The listing builds one solid part. Answer for the finished solid, in the listing's coordinates (mm). Face numbers are marked on the shaded views. A direction names the side the tool comes from. Coordinates: 2 decimals unless noted, no trailing zeros. Order: outer loops, then holes, each group sorted by start corner. A loop starts at its lowest first (then second) coordinate and runs counter-clockwise, first axis right, second up. Notation, with made-up numbers: M -16.75,-28 L 33.25,-28 A16 ccw 33.25,-9 Z; hole C -1,-16 d6. An arc over 180 degrees is marked long. One line per item, written item: value. Start each with the question number.
Q1. Each of these flat-tipped pins is pushed along its axis until it touches: pin 1 Ø11.5 at (x, z) = (-63.5, 63.5) entering from -Y (3 decimals); pin 2 Ø4 at (x, y) = (-75.5, -5.5) entering from +Z (3 decimals); pin 3 Ø15 at (y, z) = (63.5, 25.4) entering from +X (3 decimals). Where does it stop, or does it pass through?
Q2. The part is cut by section C-C on x = -63.5. Give the vertices of the cut face in (y, z) (3 decimals), then the cut area to 3 significant figures.
Q3. Straight lines are drawn through the part: line 1 along X through (y, z) = (-120, 63); line 2 along Y through (x, z) = (-113, 47) (3 decimals); line 3 along X through (y, z) = (-81, 81) (3 decimals). For each, find the intervals that lie inside material, in ascending order. Write a range as [from, to].
Q4. The part is cut by section B-B on z = 25.4. Give the vertices of the cut face in (x, y) (3 decimals), then the cut area to 3 significant figures.
Q5. Determine the mould class of the marked faces 4, 5, 6 and 7 for opening direction X: pulls with the +X half, pulls with the -X half, needs draft (parallel to the pull), parting line crosses it, or undercut.
Q6. The part is cut by section D-D on z = 127.5. Give the vertices of the cut face in (x, y) (3 decimals).
Q7. The part is cut by section A-A on y = 63.5. Give the vertices of the cut face in (x, z) (3 decimals), then the cut area to 3 significant figures.
Q8. For the marked faces 1, 2 and 3, determine the directions among +Z, -Z, +X, -X, +Y, -Y from which every point of the face is accessible in a straight line to the end or side of a thin tool.
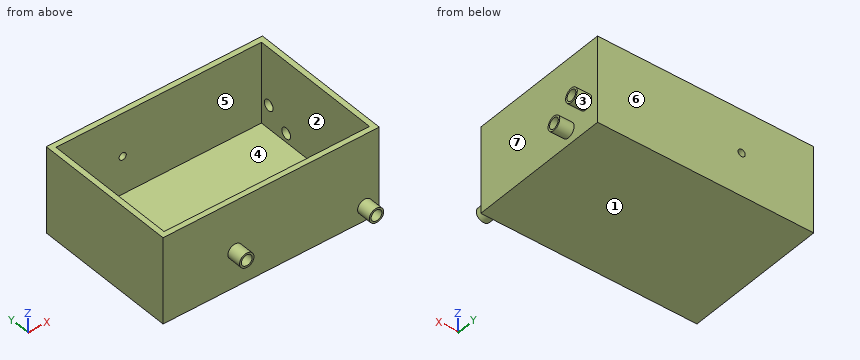
```python
from build123d import *

# Parameters (mm, degrees)
F0_W      = 381
F0_H      = 254
F1_DEPTH  = 152.4
F2_T      = -9.525
F3_R      = 12.7
F3_R_2    = 9.525
F4_DEPTH  = 25.4
F5_R      = 9.525
F6_DEPTH  = 9.525
F7_R      = 12.7
F7_R_2    = 9.525
F8_DEPTH  = 25.4
F9_R      = 9.525
F10_DEPTH = 9.525
F11_R     = 6.35
F12_DEPTH = 25.4


with BuildPart() as f1:
    # F0 (on Top) → F1 (new body)
    with BuildSketch(Plane.XY):
        Rectangle(F0_W, F0_H)
    extrude(amount=F1_DEPTH)

    # F2
    f2_openings = [f1.faces().sort_by_distance(p)[0] for p in [
        (0, 0, 152.4),
    ]]
    offset(amount=F2_T, openings=f2_openings)

    # F3 (on face) → F4 (join)
    with BuildSketch(Plane.YZ.offset(190.5)):
        with Locations((63.5, 25.4)):
            Circle(F3_R)
        with Locations((63.5, 25.4)):
            Circle(F3_R_2, mode=Mode.SUBTRACT)
        with Locations((101.6, 50.8)):
            Circle(F3_R)
        with Locations((101.6, 50.8)):
            Circle(F3_R_2, mode=Mode.SUBTRACT)
    extrude(amount=F4_DEPTH)

    # F5 (on face) → F6 (cut, through all)
    with BuildSketch(Plane.YZ.offset(190.5)):
        with Locations((63.5, 25.4)):
            Circle(F5_R)
        with Locations((101.6, 50.8)):
            Circle(F5_R)
    extrude(amount=-F6_DEPTH, mode=Mode.SUBTRACT)

    # F7 (on face) → F8 (join)
    with BuildSketch(Plane.XZ.offset(127)):
        with Locations((-63.5, 63.5)):
            Circle(F7_R)
        with Locations((-63.5, 63.5)):
            Circle(F7_R_2, mode=Mode.SUBTRACT)
        with Locations((165.1, 25.4)):
            Circle(F7_R)
        with Locations((165.1, 25.4)):
            Circle(F7_R_2, mode=Mode.SUBTRACT)
    extrude(amount=F8_DEPTH)

    # F9 (on face) → F10 (cut, through all)
    with BuildSketch(Plane.XZ.offset(127)):
        with Locations((-63.5, 63.5)):
            Circle(F9_R)
        with Locations((165.1, 25.4)):
            Circle(F9_R)
    extrude(amount=-F10_DEPTH, mode=Mode.SUBTRACT)

    # F11 (on face) → F12 (cut)
    with BuildSketch(Plane.XZ.offset(-117.475)):
        with Locations((-63.5, 76.2)):
            Circle(F11_R)
    extrude(amount=-F12_DEPTH, mode=Mode.SUBTRACT)


solid = f1.part
```
Output:
1. pin 1: stops at y = 117.475
1. pin 2: stops at z = 9.525
1. pin 3: stops at x = -180.975
2. outline: M -152.4,50.8 L -127,50.8 L -127,0 L 127,0 L 127,69.85 L 117.475,69.85 L 117.475,9.525 L -117.475,9.525 L -117.475,53.975 L -152.4,53.975 Z; M -152.4,73.025 L -117.475,73.025 L -117.475,152.4 L -127,152.4 L -127,76.2 L -152.4,76.2 Z; M 117.475,82.55 L 127,82.55 L 127,152.4 L 117.475,152.4 Z
2. area: 5,000 mm^2
3. line 1: x = [-190.5, -73.01], [-53.99, 190.5]
3. line 2: y = [-127, -117.475], [117.475, 127]
3. line 3: x = [-190.5, -180.975], [180.975, 190.5]
4. outline: M -190.5,-127 L 152.4,-127 L 152.4,-152.4 L 155.575,-152.4 L 155.575,-117.475 L -180.975,-117.475 L -180.975,117.475 L 180.975,117.475 L 180.975,73.025 L 215.9,73.025 L 215.9,76.2 L 190.5,76.2 L 190.5,127 L -190.5,127 Z; M 174.625,-152.4 L 177.8,-152.4 L 177.8,-127 L 190.5,-127 L 190.5,50.8 L 215.9,50.8 L 215.9,53.975 L 180.975,53.975 L 180.975,-117.475 L 174.625,-117.475 Z
4. area: 11,700 mm^2
5. face 4: undercut
5. face 5: undercut
5. face 6: needs draft
5. face 7: pulls with the +X half
6. outline: M -190.5,-127 L 190.5,-127 L 190.5,127 L -190.5,127 Z; hole M -180.975,-117.475 L 180.975,-117.475 L 180.975,117.475 L -180.975,117.475 Z
7. outline: M -190.5,0 L 190.5,0 L 190.5,12.7 L 215.9,12.7 L 215.9,15.875 L 180.975,15.875 L 180.975,9.525 L -180.975,9.525 L -180.975,152.4 L -190.5,152.4 Z; M 180.975,34.925 L 215.9,34.925 L 215.9,38.1 L 190.5,38.1 L 190.5,152.4 L 180.975,152.4 Z
7. area: 6,330 mm^2
8. face 1: -Z, +X, -X, +Y, -Y
8. face 2: +Z
8. face 3: +X
